```python
from build123d import *

# Parameters (mm, degrees)
SCHIZZO1_W                   = 49
SCHIZZO1_H                   = 36
ESTRUSIONE_ESTRUSIONE1_DEPTH = 144
RACCORDO1_R                  = 10


with BuildPart() as part:
    # Schizzo1 → Estrusione-Estrusione1 (new body)
    with BuildSketch(Plane.XY):
        Rectangle(SCHIZZO1_W, SCHIZZO1_H)
    extrude(amount=ESTRUSIONE_ESTRUSIONE1_DEPTH)

    # Raccordo1
    raccordo1_edges = [part.edges().sort_by_distance(p)[0] for p in [
        (0, -18, 144),
        (0, -18, 0),
        (0, 18, 0),
        (0, 18, 144),
    ]]
    fillet(raccordo1_edges, radius=RACCORDO1_R)


solid = part.part
```
Verification items for the finished model (mm, model axes). Coordinates: 2 decimals unless noted, no trailing zeros. Loops run counter-clockwise (first coordinate to the right, second up) from the corner with the lowest first, then second, coordinate; pieces in that order, holes last. Notation, with made-up numbers: (-38.5, 21.25) - (1.5, 21.25) arc R9 cw to (1.5, 30.25) - close; hole circle Ø8 at (18, -21.75). An arc over 180 degrees is marked (long way). Put each result on its own line as item: value.
Item 1: Scan lines: line 1 along Z through (x, y) = (5.5, 13); line 2 along Z through (x, y) = (-15, -16); line 3 along Y through (x, z) = (-3, 137). Record each from-to range of solid material in increasing order.
Conclusion:
line 1: z = 1.34 to 142.66
line 2: z = 4 to 140
line 3: y = -17.54 to 17.54
Item 2: Section check B-B (y = -14.5). Enter the section's corners in (x, z).
Conclusion:
outline: (-24.5, 2.4) - (24.5, 2.4) - (24.5, 141.6) - (-24.5, 141.6) - close
Item 3: Section check A-A (x = -17.5). Enter the section's corners in (y, z).
Conclusion:
outline: (-18, 10) arc R10 ccw to (-8, 0) - (8, 0) arc R10 ccw to (18, 10) - (18, 134) arc R10 ccw to (8, 144) - (-8, 144) arc R10 ccw to (-18, 134) - close
